from build123d import *

# Parameters (mm, degrees)
SKETCH1_R           = 7
BOSS_EXTRUDE1_DEPTH = 13.2
HOLE1_D             = 2
HOLE1_DEPTH         = 30
HOLE2_D             = 2
HOLE2_DEPTH         = 30
BOSS_EXTRUDE2_DEPTH = 1.5
CHAMFER1_SIZE       = 1


with BuildPart() as part:
    # Sketch1 → Boss-Extrude1 (new body)
    with BuildSketch(Plane.XY):
        with BuildLine():
            Line((-14, 0), (-14, 5))
            Line((-14, 5), (-10, 5))
            Line((-10, 5), (-10, 17))
            ThreePointArc((-10, 17), (-8.139410298, 22.809475019), (-3.25, 26.45714016))
            Line((-3.25, 26.45714016), (-3.25, 29.65714016))
            Line((-3.25, 29.65714016), (-0.25, 29.65714016))
            Line((-0.25, 29.65714016), (-0.25, 26.996874512))
            ThreePointArc((-0.25, 26.996874512), (0, 27), (0.25, 26.996874512))
            Line((0.25, 26.996874512), (0.25, 29.65714016))
            Line((0.25, 29.65714016), (3.25, 29.65714016))
            Line((3.25, 29.65714016), (3.25, 26.45714016))
            ThreePointArc((3.25, 26.45714016), (8.139410298, 22.809475019), (10, 17))
            Line((10, 17), (10, 5))
            Line((10, 5), (14, 5))
            Line((14, 5), (14, 0))
            Line((14, 0), (7, 0))
            Line((7, 0), (7, 9.858571571))
            ThreePointArc((7, 9.858571571), (0, 7), (-7, 9.858571571))
            Line((-7, 9.858571571), (-7, 0))
            Line((-7, 0), (-14, 0))
        make_face()
        with Locations((0, 17)):
            Circle(SKETCH1_R, mode=Mode.SUBTRACT)
    extrude(amount=BOSS_EXTRUDE1_DEPTH)

    # Hole1
    with Locations(Plane(origin=(3.25, 0, 0), x_dir=(0, 0, -1), z_dir=(1, 0, 0))):
        with Locations((-11.2, 27.85714016), (-2, 27.85714016), (-6.6, 27.85714016)):
            Hole(HOLE1_D / 2, depth=HOLE1_DEPTH)

    # Hole2
    with Locations(Plane(origin=(0, 5, 0), x_dir=(1, 0, 0), z_dir=(0, 1, 0))):
        with Locations((12, -2.8), (12, -10.4)):
            hole2 = Hole(HOLE2_D / 2, depth=HOLE2_DEPTH)

    # Mirror1: Hole2 across plane
    add(hole2.mirror(Plane(origin=(0, 0, 0), x_dir=(0, 0, 1), z_dir=(1, 0, 0))), mode=Mode.SUBTRACT)

    # Sketch6 → Boss-Extrude2 (add, symmetric)
    with BuildSketch(Plane.XY.offset(6.6)):
        Polygon((10, 17), (14, 5), (10, 5), align=None)
    boss_extrude2 = extrude(amount=BOSS_EXTRUDE2_DEPTH, both=True)

    # Mirror2: Boss-Extrude2 across plane
    add(boss_extrude2.mirror(Plane(origin=(0, 0, 0), x_dir=(0, 0, 1), z_dir=(1, 0, 0))))

    # Chamfer1
    chamfer1_edges = [part.edges().sort_by_distance(p)[0] for p in [
        (7, 0, 6.6),
        (-7, 0, 6.6),
    ]]
    chamfer(chamfer1_edges, length=CHAMFER1_SIZE)


solid = part.part
Design review of the part built by this model. Coordinates are the model's own, in mm. A direction names the side the tool comes from. Give positions to 0.01 mm unless a question says otherwise; leave off trailing zeros. Loops run counter-clockwise (first coordinate to the right, second up) from the corner with the lowest first, then second, coordinate; pieces in that order, holes last. Notation, with made-up numbers: (53, 26.5) -> (82, 26.5) arc R24 cw to (82, 51.5) -> close; hole circle Ø6 at (49, 30.25). An arc over 180 degrees is marked (long way). One line per question, with ' | ' between items. Start each with the question number.
(1) Insertion check: P1, Ø2, axis at x = 12, y = 12, coming from the +Z side; P2, Ø3, axis at x = -3.5, z = 6.5, coming from the +Y side; P3, Ø2.5, axis at x = -12, z = 2.8, coming from the +Y side; P4, Ø1.2, axis at x = -12.5, y = 9.5, coming from the -Z side. Each pin has a flat end and moves straight along its axis. Give the tip position at first contact, or say it passes through.
(2) For line 1 (Y direction, x = 0.75, z = 6.6); line 2 (X direction, y = 4.5, z = 11.25); line 3 (Y direction, x = 0, z = 3.25), list the stretches that pass through material, from the lowest coordinate up.
(3) Draft analysis for pull direction Z (two halves, no side actions). For faces 1 (the face through (11, 8, 8.1)), 2 (the face through (-0.05, 26.88, 10.98)), 3 (the face through (-14, 2, 7)), 4 (the face through (11, 8, 5.1)), state which applies: +Z half, -Z half, draft (parallel to the pull), parting line (faces both ways), or undercut.
(4) We need section B-B (z = 4.5). State the section outline as (x, y) points, and give its area (3 significant figures).
(5) We need section A-A (z = 6.6). State the section outline as (x, y) points.
(6) For faces 5 (the face through (0.25, 29, 7)), 6 (the face through (3.25, 29, 7)), 7 (the face through (13, 5, 2)), list the 3-axis set-ups (+Z, -Z, +X, -X, +Y, -Y) from which the entire face can be reached by the end or side of a thin tool; tool diameter is ignored.
(7) We need section C-C (x = 12). State the section outline as (y, z) points.
The answers:
1) P1: stops at z = 8.1 | P2: stops at y = 29.66 | P3: stops at y = 5 | P4: stops at z = 5.1
2) line 1: y = 7.03 to 10.04, 23.96 to 26.86, 28.86 to 29.66 | line 2: x = -14 to -12.53, -11.47 to -7, 7 to 11.47, 12.53 to 14 | line 3: y = 7 to 10, 24 to 27
3) face 1: +Z half | face 2: undercut | face 3: draft | face 4: -Z half
4) outline: (-14, 0) -> (-8, 0) -> (-7, 1) -> (-7, 9.86) arc R10 ccw to (7, 9.86) -> (7, 1) -> (8, 0) -> (14, 0) -> (14, 5) -> (10, 5) -> (10, 17) arc R10 ccw to (3.25, 26.46) -> (3.25, 29.66) -> (0.25, 29.66) -> (0.25, 27) arc R10 ccw to (-0.25, 27) -> (-0.25, 29.66) -> (-3.25, 29.66) -> (-3.25, 26.46) arc R10 ccw to (-10, 17) -> (-10, 5) -> (-14, 5) -> close; hole circle Ø14 at (0, 17) | area: 289 mm^2
5) outline: (-14, 0) -> (-8, 0) -> (-7, 1) -> (-7, 9.86) arc R10 ccw to (7, 9.86) -> (7, 1) -> (8, 0) -> (14, 0) -> (14, 5) -> (10, 17) arc R10 ccw to (3.25, 26.46) -> (3.25, 26.86) -> (-3.25, 26.86) -> (-3.25, 26.46) arc R10 ccw to (-10, 17) -> (-14, 5) -> close; (-3.25, 28.86) -> (-0.25, 28.86) -> (-0.25, 29.66) -> (-3.25, 29.66) -> close; (0.25, 28.86) -> (3.25, 28.86) -> (3.25, 29.66) -> (0.25, 29.66) -> close; hole circle Ø14 at (0, 17)
6) face 5: +Z, -Z, +Y | face 6: +Z, -Z, +X, +Y | face 7: -Z, +X, +Y
7) outline: (0, 0) -> (5, 0) -> (5, 1.8) -> (0, 1.8) -> close; (0, 3.8) -> (5, 3.8) -> (5, 5.1) -> (11, 5.1) -> (11, 8.1) -> (5, 8.1) -> (5, 9.4) -> (0, 9.4) -> close; (0, 11.4) -> (5, 11.4) -> (5, 13.2) -> (0, 13.2) -> close
